Study the drawing (mm; zero at the part's minimum x, y, z) and answer. Round coordinates to 2 decimals unless told otherwise and drop trailing zeros. Write each loop counter-clockwise with the first axis right and the second up, starting at its lowest first coordinate (ties: lowest second). Pieces come first, ordered by that corner, then holes.
(1) A cutting plane is placed at C-C, the plane x = 8.5. Give the vertices of the cut face in (y, z), and give its area (3 significant figures).
(2) A cutting plane is placed at A-A, the plane y = 10.5. Give the vertices of the cut face in (x, z).
(3) The mould has two halves that part along Z. Classify the marked faces 1 and 2: +Z half, -Z half, draft (parallel to the pull), parting line (faces both ways), or undercut.
(4) Each of these flat-tipped pins is pushed along its axis until it touches: pin 1 Ø4 at (x, z) = (20.5, 18) entering from -Y; pin 2 Ø2 at (x, z) = (8, 18) entering from -Y; pin 3 Ø3 at (x, z) = (12, 13) entering from -Y. Where does it stop, or does it pass through?
(5) Find the intervals of material crossed by probe 1 along Y at (x, z) = (10, 10.5); probe 2 along Z at (x, y) = (10.25, 2.25); probe 3 along Y at (x, z) = (2, 8.5), in increasing order.
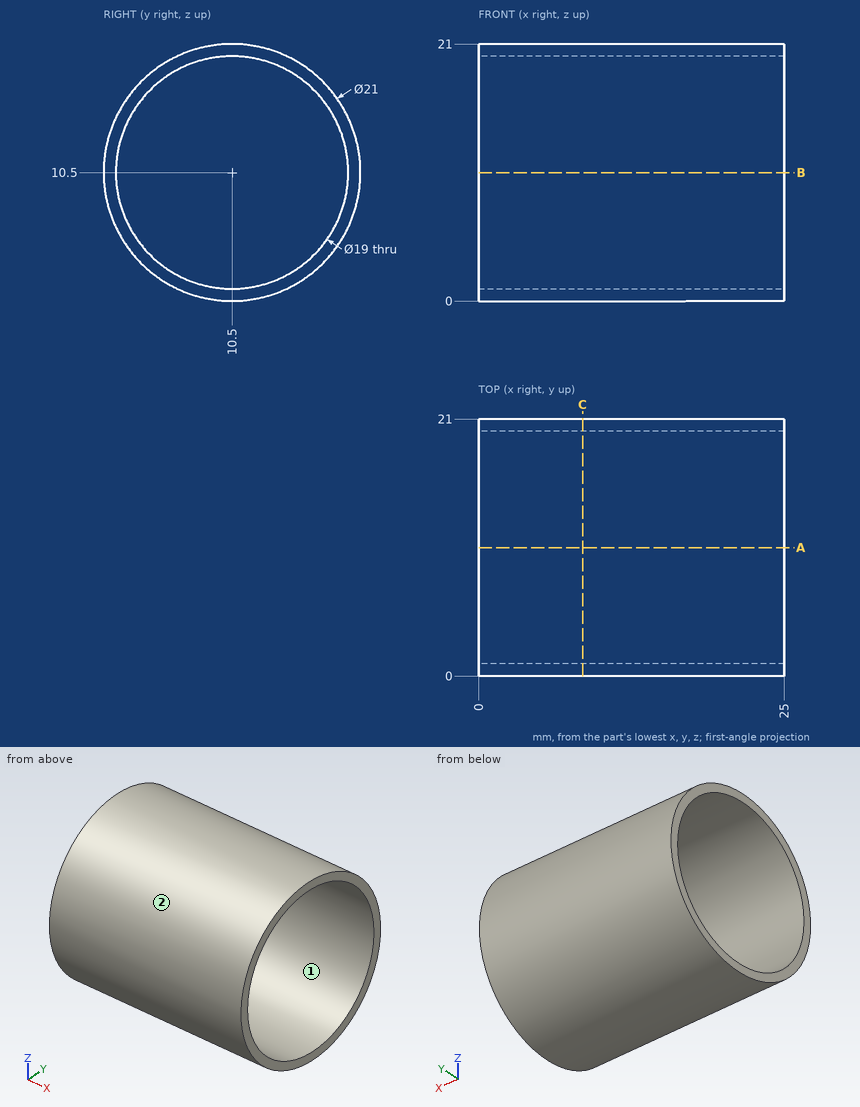
Solutions:
1. outline: circle Ø21 at (10.5, 10.5); hole circle Ø19 at (10.5, 10.5)
1. area: 62.8 mm2
2. outline: (0, 0) - (25, 0) - (25, 1) - (0, 1) - close; (0, 20) - (25, 20) - (25, 21) - (0, 21) - close
3. face 1: undercut
3. face 2: parting line
4. pin 1: stops at y = 1.56
4. pin 2: stops at y = 2.25
4. pin 3: stops at y = 0.05
5. probe 1: y = 0 to 1, 20 to 21
5. probe 2: z = 4 to 5.79, 15.21 to 17
5. probe 3: y = 0.19 to 1.21, 19.79 to 20.81
